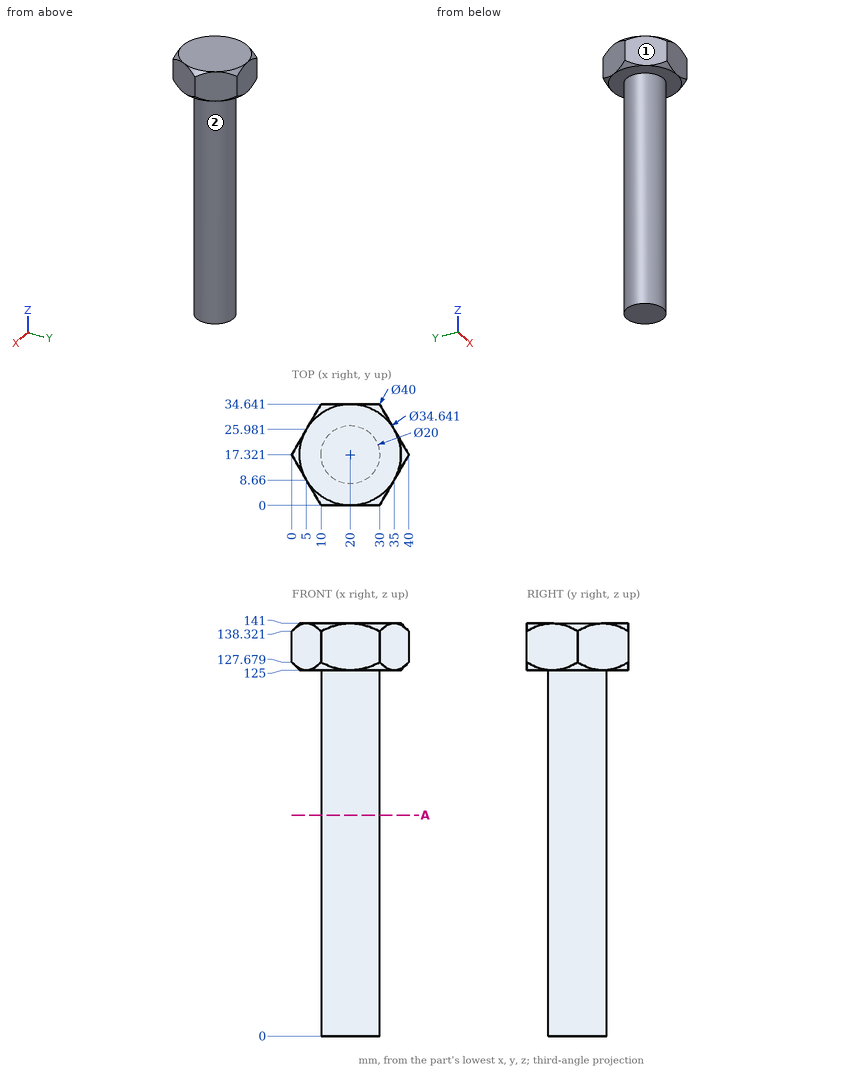
The drawing under review shows one solid part. Ordinate dimensions are in mm from its lowest x, y, z. A direction names the side the tool comes from. Give positions to 0.01 mm unless a question says otherwise; leave off trailing zeros. Order: outer loops, then holes, each group sorted by start corner. A loop starts at its lowest first (then second) coordinate and runs counter-clockwise, first axis right, second up. Notation, with made-up numbers: M 83.5,-8 L 136.5,-8 A17 cw 136.5,16 Z; hole C 13.25,49 d8. An arc over 180 degrees is marked long. One line per question, with ' | ' between items. Start each with the question number.
Q1. Machinability: for the marked faces 1 and 2, which of the approach directions +Z, -Z, +X, -X, +Y, -Y give a long, thin tool a straight path to every point of the face, cutting with its end or side? Answer none if there is none.
Q2. For pin 1 Ø1.5 at (x, y) = (33.5, 8) entering from -Z; pin 2 Ø8 at (x, z) = (18, 114.5) entering from +Y; pin 3 Ø8 at (x, z) = (13, 52) entering from -Y; pin 4 Ø6 at (x, z) = (6.5, 50) entering from -Y, all flat-tipped, find the tip position at first contact; note any pin that passes through.
Q3. For L1, parallel to Z at x = 31, y = 23.5; L2, parallel to X at y = 18, z = 41.5; L3, parallel to Y at x = 28, z = 97, list the stretches that pass through material, from the lowest coordinate up. Write a range as [from, to].
Q4. We need section A-A (z = 75.5). Write out the cut boundary in (x, y), plus the area to 3 significant figures.
Returned:
1) face 1: +Z, -Z, -X, -Y | face 2: -Z
2) pin 1: z = 125 | pin 2: y = 27.32 | pin 3: y = 7.78 | pin 4: through
3) L1: [125, 141] | L2: [10.02, 29.98] | L3: [11.32, 23.32]
4) outline: C 20,17.32 d20 | area: 314 mm2
